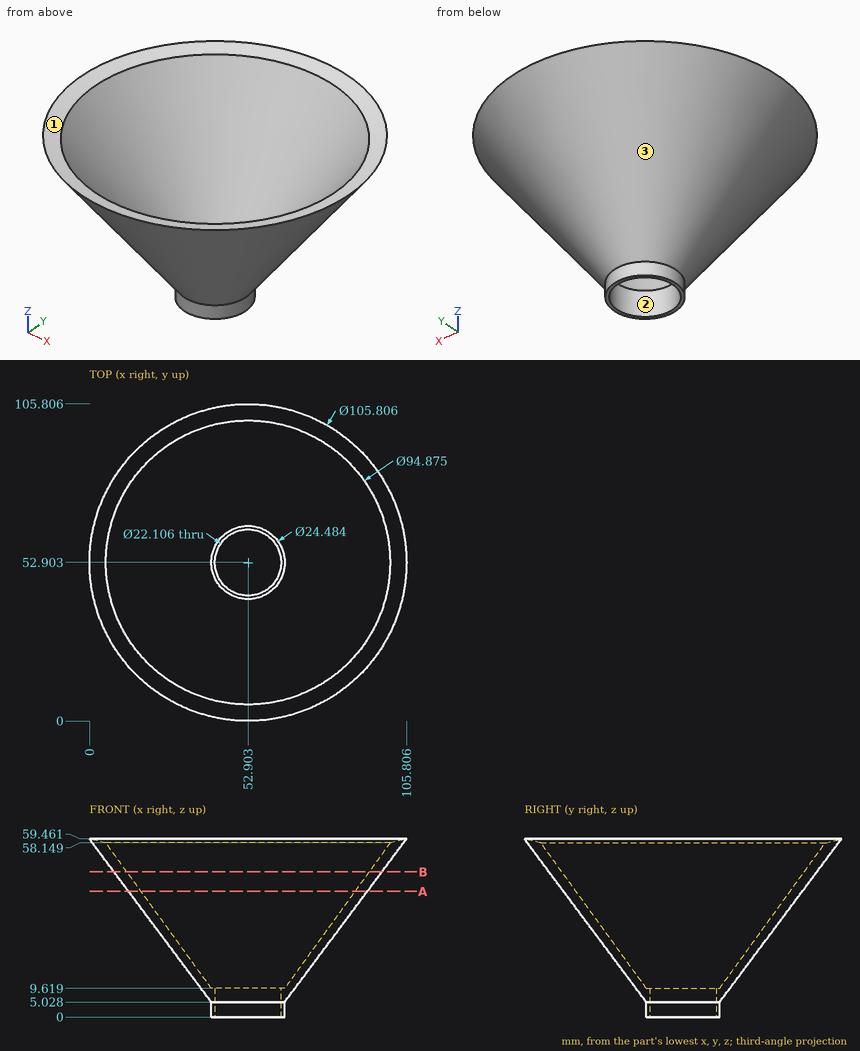
Study the drawing (mm; zero at the part's minimum x, y, z) and answer. Give positions to 0.01 mm unless a question says otherwise; leave off trailing zeros. Order: outer loops, then holes, each group sorted by start corner. A loop starts at its lowest first (then second) coordinate and runs counter-clockwise, first axis right, second up. Notation, with made-up numbers: (-35, 50) - (-25, 50) arc R22 cw to (-25, 73) - close; hole circle Ø5 at (33, 84.5). An arc over 180 degrees is marked (long way). Answer in a Markdown table with one row per item. Add a question column.
Q1. For a pull along Y with two mould halves and no side action, classify the marked faces 1, 2 and 3 as released by +Y, released by -Y, zero draft, split by the parting line, or undercut.
Q2. The part is cut by section B-B (z = 48.5). Determine the outline of the cut face in (x, y) (1 decimal).
Q3. The part is cut by section A-A (z = 42). Determine the outline of the cut face in (x, y) (1 decimal).
Q4. Given P1, Ø5, axis at y = 82.5, z = 40.5, coming from the -X side (1 decimal); P2, Ø6, axis at x = 51.5, z = 52, coming from the -Y side; P3, Ø12, axis at x = 41, y = 31, coming from the -Z side, each flat-ended and moving along its own axis, determine where each tip first touches the part or whether it passes through.
Q5. Find the intervals of material crossed by line 1 along Y through (x, z) = (81, 54) (1 decimal); line 2 along X through (y, z) = (50, 10) (1 decimal); line 3 along Y through (x, z) = (55, 22) (1 decimal), in increasing order. Write a range as [from, to].
Determined:
| question | item | result |
|---|---|---|
| 1 | face 1 | undercut |
| 1 | face 2 | undercut |
| 1 | face 3 | split by the parting line |
| 2 | outline | circle Ø89.4 at (52.9, 52.9); hole circle Ø80.9 at (52.9, 52.9) |
| 3 | outline | circle Ø79.7 at (52.9, 52.9); hole circle Ø71.5 at (52.9, 52.9) |
| 4 | P1 | stops at x = 24.1 |
| 4 | P2 | stops at y = 3.35 |
| 4 | P3 | stops at z = 13.98 |
| 5 | line 1 | y = [13, 18.5], [87.3, 92.8] |
| 5 | line 2 | x = [37.2, 40.7], [65.1, 68.6] |
| 5 | line 3 | y = [28.1, 31.8], [74, 77.7] |
